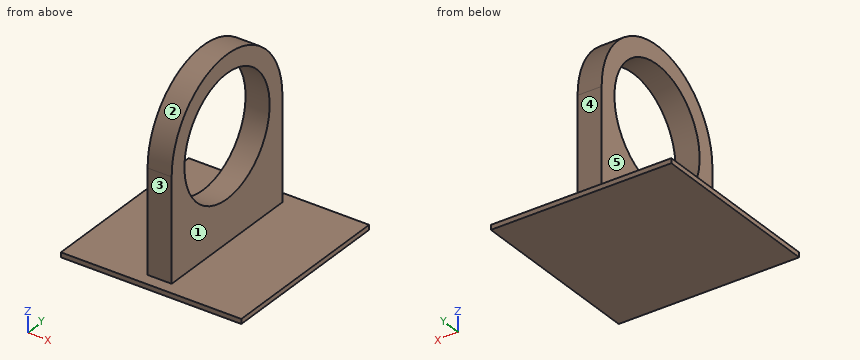
from build123d import *

# Parameters (mm, degrees)
SKETCH2_W           = 19.05
SKETCH2_H           = 19.05
BOSS_EXTRUDE1_DEPTH = 0.508
SKETCH3_W           = 2.54
SKETCH3_H           = 16.51
BOSS_EXTRUDE2_DEPTH = 19.05
CUT_EXTRUDE1_REACH  = 26.285
SKETCH4_R           = 6.35
CUT_EXTRUDE2_START  = -2.54
CUT_EXTRUDE2_DEPTH  = 2.54


with BuildPart() as part:
    # Sketch2 → Boss-Extrude1 (new body)
    with BuildSketch(Plane.XY):
        Rectangle(SKETCH2_W, SKETCH2_H)
    extrude(amount=BOSS_EXTRUDE1_DEPTH)

    # Sketch3 → Boss-Extrude2 (add)
    with BuildSketch(Plane.XY.offset(0.508)):
        Rectangle(SKETCH3_W, SKETCH3_H)
    extrude(amount=BOSS_EXTRUDE2_DEPTH)

    # Sketch4 → Cut-Extrude1 (cut, up to next)
    with BuildSketch(Plane(origin=(1.27, 0, 0), x_dir=(0, 0, -1), z_dir=(1, 0, 0)), mode=Mode.PRIVATE) as cut_extrude1_sk1:
        with Locations((-11.303, 0)):
            Circle(SKETCH4_R)
    cut_extrude1_tool1 = extrude(cut_extrude1_sk1.sketch, amount=-CUT_EXTRUDE1_REACH, mode=Mode.PRIVATE) & part.part
    add(cut_extrude1_tool1.solids().sort_by_distance((1.27, 0, 11.303))[0], mode=Mode.SUBTRACT)

    # Sketch9 → Cut-Extrude2 (cut)
    with BuildSketch(Plane(origin=(1.27, 0, 0), x_dir=(0, 0, -1), z_dir=(1, 0, 0)).offset(CUT_EXTRUDE2_START)):
        with BuildLine():
            ThreePointArc((-11.303, 12.7), (-24.003, 0), (-11.303, -12.7))
            ThreePointArc((-11.303, -12.7), (-9.0805, -10.4775), (-11.303, -8.255))
            ThreePointArc((-11.303, -8.255), (-19.558, 0), (-11.303, 8.255))
            ThreePointArc((-11.303, 8.255), (-9.0805, 10.4775), (-11.303, 12.7))
        make_face()
    extrude(amount=CUT_EXTRUDE2_DEPTH, mode=Mode.SUBTRACT)


solid = part.part
Read the model definition and answer for the solid it produces. Units are mm, in the model's axes. Face numbers are marked on the shaded views. A direction names the side the tool comes from. Coordinates: 2 decimals unless noted, no trailing zeros. Loops run counter-clockwise (first coordinate to the right, second up) from the corner with the lowest first, then second, coordinate; pieces in that order, holes last. Notation, with made-up numbers: (-35, 46.25) -> (1, 46.25) arc R12 cw to (1, 67.25) -> close; hole circle Ø11 at (-4.5, 89). An arc over 180 degrees is marked (long way). Answer in a Markdown table with one row per item.
Item 1: A cutting plane is placed at A-A on x = 0.5. Determine the outline of the cut face in (y, z) (3 decimals).
Returned:
| item | result |
|---|---|
| outline | (-9.525, 0) -> (9.525, 0) -> (9.525, 0.508) -> (8.255, 0.508) -> (8.255, 11.303) arc R8.255 ccw to (-8.255, 11.303) -> (-8.255, 0.508) -> (-9.525, 0.508) -> close; hole circle Ø12.7 at (0, 11.303) |
Item 2: A cutting plane is placed at D-D on z = 10.75. Determine the outline of the cut face in (x, y) (3 decimals), plus the area to 3 significant figures.
Returned:
| item | result |
|---|---|
| outline | (-1.27, -8.255) -> (1.27, -8.255) -> (1.27, -6.326) -> (-1.27, -6.326) -> close; (-1.27, 6.326) -> (1.27, 6.326) -> (1.27, 8.255) -> (-1.27, 8.255) -> close |
| area | 9.80 mm^2 |
Item 3: A cutting plane is placed at C-C on z = 15.75. Determine the outline of the cut face in (x, y), plus the area to 3 significant figures.
Returned:
| item | result |
|---|---|
| outline | (-1.27, -6.95) -> (1.27, -6.95) -> (1.27, -4.53) -> (-1.27, -4.53) -> close; (-1.27, 4.53) -> (1.27, 4.53) -> (1.27, 6.95) -> (-1.27, 6.95) -> close |
| area | 12.3 mm^2 |
Item 4: Each of these flat-tipped pins is pushed along its axis until it touches: P1, Ø1.3, axis at x = 0, z = 6, coming from the -Y side (3 decimals); P2, Ø1.5, axis at x = 1, z = 17.5, coming from the -Y side; P3, Ø5, axis at x = 3.5, z = 10, coming from the +Y side (3 decimals). Where does it stop, or does it pass through?
Returned:
| item | result |
|---|---|
| P1 | stops at y = -8.255 |
| P2 | stops at y = -6.2 |
| P3 | stops at y = 8.255 |
Item 5: Straight lines are drawn through the part: line 1 along Z through (x, y) = (-0.5, 0.25); line 2 along Z through (x, y) = (1.5, -2.5); line 3 along Y through (x, z) = (0, 16). For each, find the intervals that lie inside material, in ascending order. Write a range as [from, to].
Returned:
| item | result |
|---|---|
| line 1 | z = [0, 4.96], [17.65, 19.55] |
| line 2 | z = [0, 0.51] |
| line 3 | y = [-6.79, -4.27], [4.27, 6.79] |
Item 6: For the marked faces 1, 2, 3, 4 and 5, determine the directions among +Z, -Z, +X, -X, +Y, -Y from which every point of the face is accessible in a straight line to the end or side of a thin tool.
Returned:
| item | result |
|---|---|
| face 1 | +Z, +X, +Y, -Y |
| face 2 | +Z, +X, -X |
| face 3 | +Z, +X, -X, -Y |
| face 4 | +Z, +X, -X, +Y |
| face 5 | +Z, -X, +Y, -Y |
Item 7: A cutting plane is placed at B-B on y = 0. Determine the outline of the cut face in (x, z) (3 decimals).
Returned:
| item | result |
|---|---|
| outline | (-9.525, 0) -> (9.525, 0) -> (9.525, 0.508) -> (1.27, 0.508) -> (1.27, 4.953) -> (-1.27, 4.953) -> (-1.27, 0.508) -> (-9.525, 0.508) -> close; (-1.27, 17.653) -> (1.27, 17.653) -> (1.27, 19.558) -> (-1.27, 19.558) -> close |
